from build123d import *

# Parameters (mm, degrees)
SKETCH1_R           = 2.5
BOSS_EXTRUDE1_DEPTH = 1
FILLET1_R           = 1.065
FILLET2_R           = 2.13


with BuildPart() as part:
    # Sketch1 → Boss-Extrude1 (new body)
    with BuildSketch(Plane.YZ):
        Polygon((-12.5, -3.25), (-12.5, -12.5), (-3.25, -12.5), (-3.25, -10.37), (-8.863862556, -10.37), (-2.873862556, -4.38), (2.873862556, -4.38), (8.863862556, -10.37), (3.25, -10.37), (3.25, -12.5), (12.5, -12.5), (12.5, -3.25), (10.37, -3.25), (10.37, -8.863862556), (4.38, -2.873862556), (4.38, 2.873862556), (10.37, 8.863862556), (10.37, 3.25), (12.5, 3.25), (12.5, 12.5), (3.25, 12.5), (3.25, 10.37), (8.863862556, 10.37), (2.873862556, 4.38), (-2.873862556, 4.38), (-8.863862556, 10.37), (-3.25, 10.37), (-3.25, 12.5), (-12.5, 12.5), (-12.5, 3.25), (-10.37, 3.25), (-10.37, 8.863862556), (-4.38, 2.873862556), (-4.38, -2.873862556), (-10.37, -8.863862556), (-10.37, -3.25), align=None)
        with Locations(Location((0, 0, 0), (0, 0, 270))):
            Circle(SKETCH1_R, mode=Mode.SUBTRACT)
    extrude(amount=BOSS_EXTRUDE1_DEPTH)

    # Fillet1
    fillet1_edges = [part.edges().sort_by_distance(p)[0] for p in [
        (0.5, -10.37, -8.863862556),
        (0.5, 2.873862556, -4.38),
        (0.5, -2.873862556, -4.38),
        (0.5, -4.38, 2.873862556),
        (0.5, -4.38, -2.873862556),
        (0.5, -2.873862556, 4.38),
        (0.5, 2.873862556, 4.38),
        (0.5, 4.38, 2.873862556),
        (0.5, 4.38, -2.873862556),
        (0.5, -8.863862556, -10.37),
        (0.5, 8.863862556, -10.37),
        (0.5, 10.37, -8.863862556),
        (0.5, -10.37, 8.863862556),
        (0.5, -8.863862556, 10.37),
        (0.5, 10.37, 8.863862556),
        (0.5, 8.863862556, 10.37),
        (0.5, 12.5, 3.25),
        (0.5, -3.25, -12.5),
        (0.5, -10.37, 3.25),
        (0.5, 10.37, 3.25),
        (0.5, -10.37, -3.25),
        (0.5, -12.5, -3.25),
        (0.5, -12.5, 3.25),
        (0.5, 3.25, -10.37),
        (0.5, -3.25, -10.37),
        (0.5, 3.25, -12.5),
        (0.5, 10.37, -3.25),
        (0.5, 12.5, -3.25),
        (0.5, 3.25, 12.5),
        (0.5, 3.25, 10.37),
        (0.5, -3.25, 10.37),
        (0.5, -3.25, 12.5),
    ]]
    fillet(fillet1_edges, radius=FILLET1_R - 0.0001)  # a hair under: the kernel refuses the full size

    # Fillet2
    fillet2_edges = [part.edges().sort_by_distance(p)[0] for p in [
        (0.5, -12.5, 12.5),
        (0.5, 12.5, 12.5),
        (0.5, 12.5, -12.5),
        (0.5, -12.5, -12.5),
    ]]
    fillet(fillet2_edges, radius=FILLET2_R)


solid = part.part
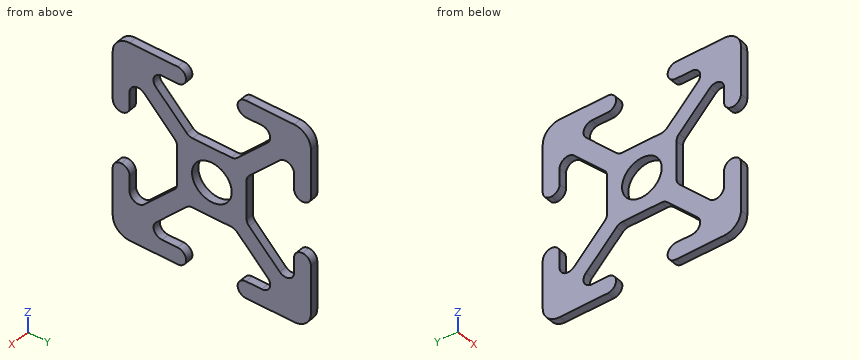
Can you work these out from the model? Positions are in its coordinate system, mm. Coordinates: 2 decimals unless noted, no trailing zeros. Order: outer loops, then holes, each group sorted by start corner. A loop starts at its lowest first (then second) coordinate and runs counter-clockwise, first axis right, second up. Notation, with made-up numbers: (-8.75, 45.25) - (7.25, 45.25) arc R21 cw to (7.25, 50.25) - close; hole circle Ø11 at (-5.75, -33.75). An arc over 180 degrees is marked (long way). Answer as a JSON object with one key per item and string values. Group by question number.
Q1. Imagine slicing it at A-A (y = 0). Please give me the cut outline in (x, z), and give its area (3 significant figures).
Q2. I need wall thicknesses on line 1 (Y direction, x = 0.3, z = 0); line 2 (Y direction, x = 0.3, z = 7); line 3 (Y direction, x = 0.4, z = -6). Which ranges of each line are inside material? Lowest first, please. Write a range as from..to.
Q3. Will these pins go through, and if not, where does the flat tip stop? P1, Ø4, axis at y = 0, z = 0, coming from the -X side; P2, Ø6, axis at y = 3.5, z = -9, coming from the +X side.
Q4. Imagine slicing it at D-D (y = 6). Please give me the cut outline in (x, z).
Q5. Imagine slicing it at C-C (z = -5.5). Please give me the cut outline in (x, y).
Determined:
{
 "1": {"outline": "(0, -4.38) - (1, -4.38) - (1, -2.5) - (0, -2.5) - close; (0, 2.5) - (1, 2.5) - (1, 4.38) - (0, 4.38) - close", "area": "3.76 mm2"},
 "2": {"line 1": "y = -4.38..-2.5, 2.5..4.38", "line 2": "y = -12.5..-10.1, -8.51..-5.49, 5.49..8.51, 10.1..12.5", "line 3": "y = -12.5..-10.37, -7.51..-4.49, 4.49..7.51, 10.37..12.5"},
 "3": {"P1": "passes through", "P2": "stops at x = 1"},
 "4": {"outline": "(0, -12.5) - (1, -12.5) - (1, -10.37) - (0, -10.37) - close; (0, -7.51) - (1, -7.51) - (1, -4.49) - (0, -4.49) - close; (0, 4.49) - (1, 4.49) - (1, 7.51) - (0, 7.51) - close; (0, 10.37) - (1, 10.37) - (1, 12.5) - (0, 12.5) - close"},
 "5": {"outline": "(0, -12.5) - (1, -12.5) - (1, -10.37) - (0, -10.37) - close; (0, -7.01) - (1, -7.01) - (1, -3.99) - (0, -3.99) - close; (0, 3.99) - (1, 3.99) - (1, 7.01) - (0, 7.01) - close; (0, 10.37) - (1, 10.37) - (1, 12.5) - (0, 12.5) - close"}
}
